Input: part model. Units: mm. Frame: model coordinates. A direction names the side the tool comes from. Coordinates: 2 decimals unless noted, no trailing zeros. Order: outer loops, then holes, each group sorted by start corner. A loop starts at its lowest first (then second) coordinate and runs counter-clockwise, first axis right, second up. Notation, with made-up numbers: (16, 9.5) - (75, 9.5) arc R11 cw to (75, 18.5) - close; hole circle Ø2 at (-14, -9). An arc over 180 degrees is marked (long way). One line per question, with ' | ' between items.
from build123d import *

# Parameters (mm, degrees)
SKETCH_1_W            = 45.23
SKETCH_1_H            = 24.73
EXTRUDE_1_DEPTH       = 28.9
SKETCH_2_R            = 2.9
EXTRUDE_2_DEPTH       = 3.4
EXTRUDE_3_DEPTH       = 1.4
SKETCH_4_R            = 0.8
CUT_EXTRUDE_1_DEPTH   = 5
SKETCH_6_R            = 0.8
CUT_EXTRUDE_2_DEPTH   = 4.1
EXTRUDE_START         = 1.5
SKETCH_7_R            = 0.8
EXTRUDE_5_DEPTH       = 1.5
EXTRUDE_6_DEPTH       = 24.73
EXTRUDE_START_2       = 3.5
SKETCH_5_R            = 2.9
EXTRUDE_4_DEPTH       = 3.5
SKETCH_11_W           = 39.736399629
SKETCH_11_H           = 38.5
SKETCH_11_W_2         = 19.736399629
SKETCH_11_H_2         = 18.5
CUT_EXTRUDE_1_2_DEPTH = 62.642240388


with BuildPart() as part:
    # 草图1 → 凸台-拉伸1 (new body)
    with BuildSketch(Plane.XY):
        with Locations((22.615, 12.365)):
            Rectangle(SKETCH_1_W, SKETCH_1_H)
    extrude(amount=EXTRUDE_1_DEPTH)

    # 草图2 → 凸台-拉伸2 (add)
    with BuildSketch(Plane.XY.offset(28.9)):
        with Locations(Location((35.115, 12.365, 0), (0, 0, 180))):
            Circle(SKETCH_2_R)
    extrude(amount=EXTRUDE_2_DEPTH)

    # 草图3 → 凸台-拉伸3 (add)
    with BuildSketch(Plane.XY.offset(28.9)):
        with BuildLine():
            Line((29.3, 21.702332328), (29.3, 24.73))
            Line((29.3, 24.73), (0, 24.73))
            Line((0, 24.73), (0, 0))
            Line((0, 0), (29.3, 0))
            Line((29.3, 0), (29.3, 3.027667672))
            ThreePointArc((29.3, 3.027667672), (24.115, 12.365), (29.3, 21.702332328))
        make_face()
    extrude(amount=EXTRUDE_3_DEPTH)

    # 草图4 → Cut-Extrude 1 (cut)
    with BuildSketch(Plane.XY.offset(30.3)):
        with Locations((5.95, 22.78)):
            Circle(SKETCH_4_R)
        with Locations((26.65, 22.78)):
            Circle(SKETCH_4_R)
        with Locations(Location((26.65, 1.95, 0), (0, 0, 180))):
            Circle(SKETCH_4_R)
        with Locations(Location((5.95, 1.95, 0), (0, 0, 180))):
            Circle(SKETCH_4_R)
    extrude(amount=-CUT_EXTRUDE_1_DEPTH, mode=Mode.SUBTRACT)

    # 草图6 → 切除-拉伸2 (cut)
    with BuildSketch(Plane(origin=(0, 0, 0), x_dir=(-1, 0, 0), z_dir=(0, 0, -1))):
        with Locations((-26.71, 22.615)):
            Circle(SKETCH_6_R)
        with Locations((-2.27, 22.615)):
            Circle(SKETCH_6_R)
        with Locations((-2.27, 2.115)):
            Circle(SKETCH_6_R)
        with Locations((-26.71, 2.115)):
            Circle(SKETCH_6_R)
    extrude(amount=-CUT_EXTRUDE_2_DEPTH, mode=Mode.SUBTRACT)

    # 草图7 → 凸台-拉伸5 (add)
    with BuildSketch(Plane(origin=(0, 0, 0), x_dir=(-1, 0, 0), z_dir=(0, 0, -1)).offset(EXTRUDE_START)):
        with BuildLine():
            Line((0, 24.73), (-29.3, 24.73))
            Line((-29.3, 24.73), (-29.3, 21.702332328))
            ThreePointArc((-29.3, 21.702332328), (-24.115, 12.365), (-29.3, 3.027667672))
            Line((-29.3, 3.027667672), (-29.3, 0))
            Line((-29.3, 0), (0, 0))
            Line((0, 0), (0, 24.73))
        make_face()
        with Locations((-26.71, 2.115)):
            Circle(SKETCH_7_R, mode=Mode.SUBTRACT)
        with Locations((-2.27, 2.115)):
            Circle(SKETCH_7_R, mode=Mode.SUBTRACT)
        with Locations((-26.71, 22.615)):
            Circle(SKETCH_7_R, mode=Mode.SUBTRACT)
        with Locations((-2.27, 22.615)):
            Circle(SKETCH_7_R, mode=Mode.SUBTRACT)
    extrude(amount=-EXTRUDE_5_DEPTH)

    # 草图10 → 凸台-拉伸6 (add, through all)
    with BuildSketch(Plane(origin=(0, 0, 0), x_dir=(1, 0, 0), z_dir=(0, 1, 0))):
        Polygon((5.2, 1.5), (5.2, 3.5), (16.6, 3.5), (18.6, 1.5), align=None)
    extrude(amount=EXTRUDE_6_DEPTH)

    # 草图5 → 凸台-拉伸4 (add)
    with BuildSketch(Plane(origin=(0, 0, 0), x_dir=(-1, 0, 0), z_dir=(0, 0, -1)).offset(EXTRUDE_START_2)):
        with Locations((-35.115, 12.365)):
            Circle(SKETCH_5_R)
    extrude(amount=-EXTRUDE_4_DEPTH)

    # 草图11 → Cut-Extrude 1 2 (cut, through all)
    with BuildSketch(Plane(origin=(0, 0, -1.5), x_dir=(-1, 0, 0), z_dir=(0, 0, -1))):
        with Locations((-9.868199815, 12.365)):
            Rectangle(SKETCH_11_W, SKETCH_11_H)
        with Locations((-9.868199815, 12.365)):
            Rectangle(SKETCH_11_W_2, SKETCH_11_H_2, mode=Mode.SUBTRACT)
    extrude(amount=CUT_EXTRUDE_1_2_DEPTH, mode=Mode.SUBTRACT)


solid = part.part
Item 1: Contact query for flat-ended pins moving along their axis: P1, Ø0.8, axis at y = 1, z = -1, coming from the +X side; P2, Ø2, axis at x = 2.27, y = 22.615, coming from the +Z side; P3, Ø0.5, axis at x = 26.5, y = 2, coming from the +Z side. Output: stop coordinate, or through.
Data:
P1: x = 29.3 | P2: z = 30.3 | P3: z = 25.3
Item 2: Ray query, line 1 (X direction, y = 1.95, z = 29.1); line 2 (X direction, y = 1.95, z = 28.45); line 3 (Z direction, x = 29.5, y = 1.25). Return the intervals inside material, ascending.
Data:
line 1: 0 to 5.15, 6.75 to 25.85, 27.45 to 29.3 | line 2: 0 to 5.15, 6.75 to 25.85, 27.45 to 45.23 | line 3: 0 to 28.9
Item 3: Section D-D on x = 26.71. Return the cut outline in (y, z) (3 decimals).
Data:
outline: (0, -1.5) - (1.315, -1.5) - (1.315, 4.1) - (2.915, 4.1) - (2.915, -1.5) - (5.269, -1.5) - (5.269, 0) - (19.461, 0) - (19.461, -1.5) - (21.815, -1.5) - (21.815, 4.1) - (23.415, 4.1) - (23.415, -1.5) - (24.73, -1.5) - (24.73, 30.3) - (23.578, 30.3) - (23.578, 25.3) - (21.982, 25.3) - (21.982, 30.3) - (19.461, 30.3) - (19.461, 28.9) - (5.269, 28.9) - (5.269, 30.3) - (2.748, 30.3) - (2.748, 25.3) - (1.152, 25.3) - (1.152, 30.3) - (0, 30.3) - close
Item 4: Section A-A on x = 12.5. Return the cut outline in (y, z) (3 decimals).
Data:
outline: (0, -1.5) - (3.115, -1.5) - (3.115, -3.5) - (21.615, -3.5) - (21.615, -1.5) - (24.73, -1.5) - (24.73, 30.3) - (0, 30.3) - close
Item 5: Draft query along X for faces 4 (the face through (2.905, 1.628, 1.261)), 5 (the face through (23, 0, 14)), 6 (the face through (29.3, 2, -1)). Return one class per face: released by +X, released by -X, zero draft, split by the parting line, or undercut.
Data:
face 4: undercut | face 5: zero draft | face 6: released by +X
Item 6: Access query for faces 1 (the face through (27, 2, 25.3)), 2 (the face through (29.3, 23, 30)), 3 (the face through (29.3, 23, -1)). Directions: +Z, -Z, +X, -X, +Y, -Y. A direction counts if a zero-diameter tool reaches every point of the face in a straight line with its end or side. Return the directions, or none.
Data:
face 1: +Z | face 2: +Z, +X, +Y, -Y | face 3: -Z, +X, +Y, -Y
Item 7: Section B-B on y = 8.5. Return the cut outline in (x, z), and give its area (3 significant figures).
Data:
outline: (0, -1.5) - (5.2, -1.5) - (5.2, -3.5) - (16.6, -3.5) - (18.6, -1.5) - (24.82, -1.5) - (24.82, 0) - (45.23, 0) - (45.23, 28.9) - (24.82, 28.9) - (24.82, 30.3) - (0, 30.3) - close | area: 1,400 mm^2
Item 8: Section C-C on x = 2.27. Return the cut outline in (y, z) (3 decimals).
Data:
outline: (0, -1.5) - (1.315, -1.5) - (1.315, 4.1) - (2.915, 4.1) - (2.915, -1.5) - (21.815, -1.5) - (21.815, 4.1) - (23.415, 4.1) - (23.415, -1.5) - (24.73, -1.5) - (24.73, 30.3) - (0, 30.3) - close
